```python
from build123d import *

# Parameters (mm, degrees)
ESBO_O1_W                   = 22.5248
ESBO_O1_H                   = 65
RESSALTO_EXTRUS_O1_DEPTH    = 12.7
ESBO_O2_W                   = 5.08
ESBO_O2_H                   = 7.62
CORTE_EXTRUS_O1_DEPTH       = 13.7
FURO_COM_FOLGA_DE_M31_D     = 3.4544
FURO_COM_FOLGA_DE_M31_DEPTH = 22.5248


with BuildPart() as part:
    # Esboço1 → Ressalto-extrusão1 (new body)
    with BuildSketch(Plane(origin=(12.7, 0, 0), x_dir=(0, 0, -1), z_dir=(1, 0, 0))):
        with Locations((-11.2624, 32.5)):
            Rectangle(ESBO_O1_W, ESBO_O1_H)
    extrude(amount=-RESSALTO_EXTRUS_O1_DEPTH)

    # Esboço2 → Corte-extrusão1 (cut, through all)
    with BuildSketch(Plane.ZY):
        with Locations((19.9848, 32.5)):
            Rectangle(ESBO_O2_W, ESBO_O2_H)
    extrude(amount=-CORTE_EXTRUS_O1_DEPTH, mode=Mode.SUBTRACT)

    # Furo com folga de M31
    with Locations(Plane(origin=(0, 0, 0), x_dir=(-1, 0, 0), z_dir=(0, 0, -1))):
        with Locations((-6.35, 12.7), (-6.35, 52.3)):
            Hole(FURO_COM_FOLGA_DE_M31_D / 2, depth=FURO_COM_FOLGA_DE_M31_DEPTH)


solid = part.part
```
The model under review builds one solid part; all positions refer to its coordinate system, in mm. A direction names the side the tool comes from. Round coordinates to 2 decimals unless told otherwise and drop trailing zeros. Loops run counter-clockwise (first coordinate to the right, second up) from the corner with the lowest first, then second, coordinate; pieces in that order, holes last. Notation, with made-up numbers: (21, 48.5) -> (59, 48.5) arc R32 ccw to (59, 79.5) -> close; hole circle Ø5 at (32, 19). An arc over 180 degrees is marked (long way). Answer as a JSON object with one key per item and string values. Group by question number.
1) For line 1 (Y direction, x = 6.35, z = 15.25); line 2 (Y direction, x = 11, z = 19.5); line 3 (Y direction, x = 7.25, z = 14), list the stretches that pass through material, from the lowest coordinate up. Write a range as [from, to].
2) We need section A-A on y = 52.3. Write out the cut boundary in (x, z).
3) For faces 1 (the face through (0, 33, 11)), 2 (the face through (6, 28.69, 20)), list the 3-axis set-ups (+Z, -Z, +X, -X, +Y, -Y) from which the entire face can be reached by the end or side of a thin tool; tool diameter is ignored.
4) We need section D-D on x = 6. Write out the cut boundary in (y, z).
5) For pin 1 Ø3 at (x, y) = (6.35, 52.3) entering from +Z; pin 2 Ø4 at (x, y) = (5.5, 33.5) entering from +Z, all flat-tipped, find the tip position at first contact; note any pin that passes through.
6) Mouldability with a two-part tool opening along Z and no side actions: class faces 3 (the face through (6, 32, 0)), 4 (the face through (6.125, 54.013, 11.42)), 5 (the face through (6, 50, 22.525)) as released by +Z, released by -Z, zero draft, split by the parting line, or undercut.
7) We need section B-B on z = 12.5. Write out the cut boundary in (x, y), then the cut area to 3 significant figures.
8) We need section C-C on x = 2.75. Write out the cut boundary in (y, z).
Result set:
{
 "1": {"line 1": "[0, 10.97], [14.43, 50.57], [54.03, 65]", "line 2": "[0, 28.69], [36.31, 65]", "line 3": "[0, 11.23], [14.17, 50.83], [53.77, 65]"},
 "2": {"outline": "(0, 0) -> (4.62, 0) -> (4.62, 22.52) -> (0, 22.52) -> close; (8.08, 0) -> (12.7, 0) -> (12.7, 22.52) -> (8.08, 22.52) -> close"},
 "3": {"face 1": "+Z, -Z, -X, +Y, -Y", "face 2": "+Z, +X, -X"},
 "4": {"outline": "(0, 0) -> (11.01, 0) -> (11.01, 22.52) -> (0, 22.52) -> close; (14.39, 0) -> (50.61, 0) -> (50.61, 22.52) -> (36.31, 22.52) -> (36.31, 17.44) -> (28.69, 17.44) -> (28.69, 22.52) -> (14.39, 22.52) -> close; (53.99, 0) -> (65, 0) -> (65, 22.52) -> (53.99, 22.52) -> close"},
 "5": {"pin 1": "through", "pin 2": "z = 17.44"},
 "6": {"face 3": "released by -Z", "face 4": "zero draft", "face 5": "released by +Z"},
 "7": {"outline": "(0, 0) -> (12.7, 0) -> (12.7, 65) -> (0, 65) -> close; hole circle Ø3.45 at (6.35, 12.7); hole circle Ø3.45 at (6.35, 52.3)", "area": "807 mm²"},
 "8": {"outline": "(0, 0) -> (65, 0) -> (65, 22.52) -> (36.31, 22.52) -> (36.31, 17.44) -> (28.69, 17.44) -> (28.69, 22.52) -> (0, 22.52) -> close"}
}
